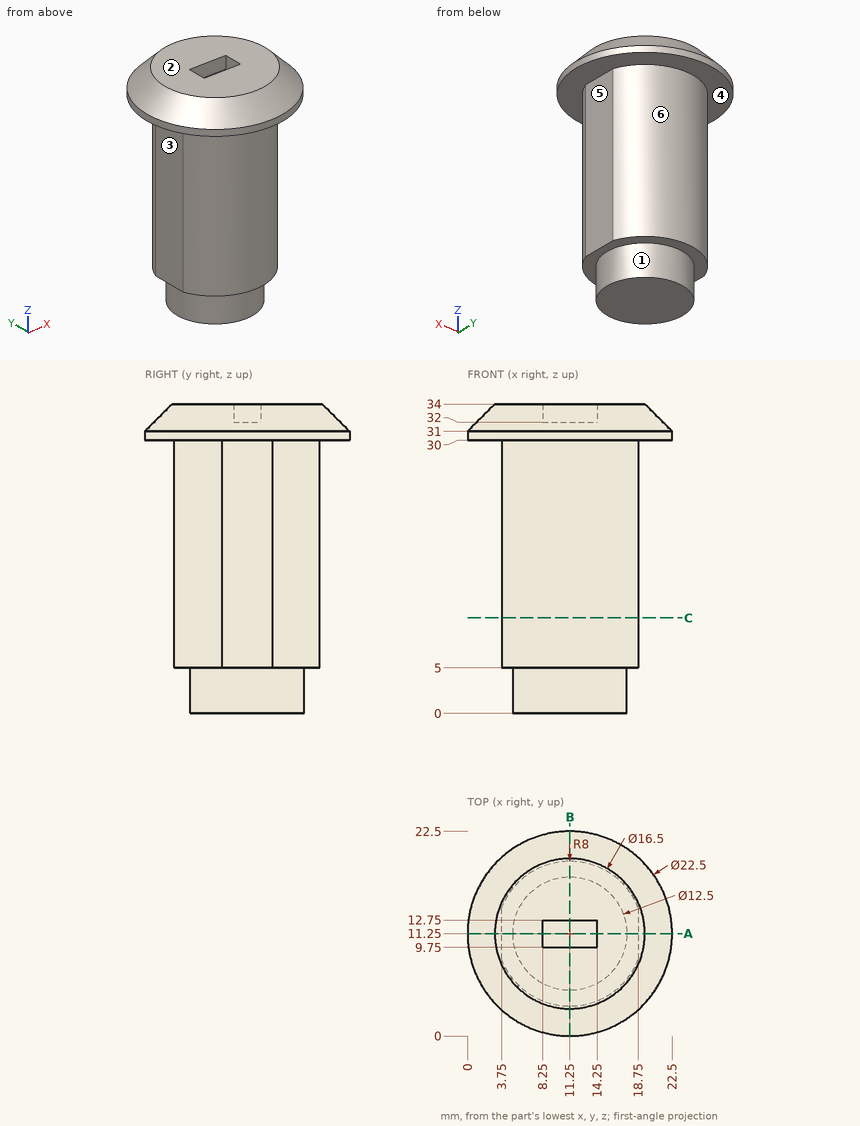
Verification items for this drawing (mm, ordinates from the low corner). A direction names the side the tool comes from. Coordinates: 2 decimals unless noted, no trailing zeros. Order: outer loops, then holes, each group sorted by start corner. A loop starts at its lowest first (then second) coordinate and runs counter-clockwise, first axis right, second up. Notation, with made-up numbers: (39, 30.25) -> (64, 30.25) arc R27 ccw to (64, 46.25) -> close; hole circle Ø2 at (-35, -8). An arc over 180 degrees is marked (long way). Put each result on its own line as item: value. Start each with the question number.
1. Cross-section at C-C, the plane z = 10.5. Record the boundary of the cut face in (x, y).
2. Cross-section at A-A, the plane y = 11.25. Record the boundary of the cut face in (x, z).
3. Access from +Z, -Z, +X, -X, +Y, -Y to the whole of each face (thin tool, end or side, straight path). Record for the marked faces 4, 5 and 6.
4. Material ranges on L1, parallel to Z at x = 17.75, y = 9; L2, parallel to X at y = 12.75, z = 15; L3, parallel to Z at x = 3, y = 17.25, recorded low to high. Write a range as [from, to].
5. Go/stop test with flat-tipped pins: pin 1 Ø8 at (y, z) = (8.5, 8) entering from -X; pin 2 Ø1.5 at (x, z) = (5.5, 29) entering from +Y (3 decimals); pin 3 Ø1.5 at (x, y) = (12.5, 11.5) entering from +Z. Record where each tip stops, or that it passes through.
6. Mould release check, pull along X, two halves, no side actions. Record for the marked faces 1, 2 and 3: released by +X, released by -X, zero draft, split by the parting line, or undercut.
7. Cross-section at B-B, the plane x = 11.25. Record the boundary of the cut face in (y, z), then the cut area to 4 significant figures.
Computed:
1. outline: (3.75, 8.47) arc R8 ccw to (18.75, 8.47) -> (18.75, 14.03) arc R8 ccw to (3.75, 14.03) -> close
2. outline: (0, 30) -> (3.75, 30) -> (3.75, 5) -> (5, 5) -> (5, 0) -> (17.5, 0) -> (17.5, 5) -> (18.75, 5) -> (18.75, 30) -> (22.5, 30) -> (22.5, 31) -> (19.5, 34) -> (14.25, 34) -> (14.25, 32) -> (8.25, 32) -> (8.25, 34) -> (3, 34) -> (0, 31) -> close
3. face 4: -Z
3. face 5: -Z, +X, +Y, -Y
3. face 6: -Z, +Y
4. L1: [5, 34]
4. L2: [3.75, 18.75]
4. L3: [30, 32.05]
5. pin 1: x = 3.75
5. pin 2: y = 17.495
5. pin 3: z = 32
6. face 1: split by the parting line
6. face 2: zero draft
6. face 3: released by -X
7. outline: (0, 30) -> (3.25, 30) -> (3.25, 5) -> (5, 5) -> (5, 0) -> (17.5, 0) -> (17.5, 5) -> (19.25, 5) -> (19.25, 30) -> (22.5, 30) -> (22.5, 31) -> (19.5, 34) -> (12.75, 34) -> (12.75, 32) -> (9.75, 32) -> (9.75, 34) -> (3, 34) -> (0, 31) -> close
7. area: 537.5 mm2
